```python
from build123d import *

# Parameters (mm, degrees)
SKETCH_1_W               = 198
SKETCH_1_H               = 30
EXTRUDE_1_DEPTH          = 2
HOLE_WIZARD_1_D          = 2.75
HOLE_WIZARD_1_DEPTH      = 100
CUT_EXTRUDE_1_DEPTH      = 101.149887668
CUT_EXTRUDE_1_DEPTH_BACK = 101.149887668


with BuildPart() as part:
    # 草图1 → 凸台-拉伸1 (new body)
    with BuildSketch(Plane(origin=(0, 0, 0), x_dir=(1, 0, 0), z_dir=(0, 1, 0))):
        Rectangle(SKETCH_1_W, SKETCH_1_H)
    extrude(amount=EXTRUDE_1_DEPTH)

    # 孔1
    with Locations(Plane(origin=(0, 2, 0), x_dir=(1, 0, 0), z_dir=(0, 1, 0))):
        with Locations((95, 10.999999819), (95, -11), (20.000000003, 10.999999819), (20.000000003, -11), (-95.2, 10.999999819), (-95.2, -11), (-20.200000003, 10.999999819), (-20.200000003, -11), (-34.700003407, -11), (-62.700003407, -11), (62.500003407, -11), (34.500003407, -11)):
            Hole(HOLE_WIZARD_1_D / 2, depth=HOLE_WIZARD_1_DEPTH)

    # 草图4 → 切除-拉伸1 (cut, two sides: drawn at the far end of the back side and taken through both)
    with BuildSketch(Plane(origin=(0, 2, 0), x_dir=(1, 0, 0), z_dir=(0, 1, 0)).offset(-CUT_EXTRUDE_1_DEPTH_BACK)):
        with BuildLine():
            Line((-10, 7), (10, 7))
            ThreePointArc((10, 7), (17, 0), (10, -7))
            Line((10, -7), (-10, -7))
            ThreePointArc((-10, -7), (-17, 0), (-10, 7))
        make_face()
        with BuildLine():
            Line((-84.999999997, 7), (-30.400000007, 7))
            ThreePointArc((-30.400000007, 7), (-23.400000007, 0), (-30.400000007, -7))
            Line((-30.400000007, -7), (-84.999999997, -7))
            ThreePointArc((-84.999999997, -7), (-91.999999997, 0), (-84.999999997, 7))
        make_face()
        with BuildLine():
            Line((84.999999997, 7), (30.400000007, 7))
            ThreePointArc((30.400000007, 7), (23.400000007, 0), (30.400000007, -7))
            Line((30.400000007, -7), (84.999999997, -7))
            ThreePointArc((84.999999997, -7), (91.999999997, 0), (84.999999997, 7))
        make_face()
    extrude(amount=CUT_EXTRUDE_1_DEPTH + CUT_EXTRUDE_1_DEPTH_BACK, mode=Mode.SUBTRACT)


solid = part.part
```
The model under review builds one solid part; all positions refer to its coordinate system, in mm. A direction names the side the tool comes from. Round coordinates to 2 decimals unless told otherwise and drop trailing zeros. Loops run counter-clockwise (first coordinate to the right, second up) from the corner with the lowest first, then second, coordinate; pieces in that order, holes last. Notation, with made-up numbers: M 37,-36 L 72,-36 A6 cw 72,-31 Z; hole C -5,-28 d1. An arc over 180 degrees is marked long. Write item = value, one per line.
Item 1: Machinability: for faces 3 (the cylindrical face through (17, 1, 0)), 4 (the flat face through (-1, 0, -10)), which of the approach directions +Z, -Z, +X, -X, +Y, -Y give a long, thin tool a straight path to every point of the face, cutting with its end or side? Answer none if there is none.
Return value:
face_3 = +Y, -Y
face_4 = +Z, -Z, +X, -X, -Y
Item 2: Take a section at B-B on y = 0.3. State how many separate pieces and enclosed holes the cut face has, then the cut area to 3 significant figures.
Return value:
separate_pieces = 1
enclosed_holes = 15
area = 3,600 mm2
Item 3: The part is to be moulded in two halves that separate along Z. For faces 1 (the flat face through (-1, 2, -10)), 2 (the cylindrical face through (92, 1, 0)), say which applies: released by +Z, released by -Z, zero draft, split by the parting line, or undercut.
Return value:
face_1 = zero draft
face_2 = undercut
Item 4: Take a section at C-C on x = -5. Write out the cut boundary in (y, z).
Return value:
outline = M 0,-15 L 2,-15 L 2,-7 L 0,-7 Z; M 0,7 L 2,7 L 2,15 L 0,15 Z
Item 5: Insertion check: P1, Ø2.5, axis at x = -34.7, z = 11, coming from the -Y side. The pin has a flat end and moves straight along its axis. Give the tip position at first contact, or say it passes through.
Return value:
P1 = through
Item 6: Take a section at A-A on z = 0. Write out the cut boundary in (x, y).
Return value:
outline = M -99,0 L -92,0 L -92,2 L -99,2 Z; M -23.4,0 L -17,0 L -17,2 L -23.4,2 Z; M 17,0 L 23.4,0 L 23.4,2 L 17,2 Z; M 92,0 L 99,0 L 99,2 L 92,2 Z
Item 7: For line 1 (Z direction, x = 81, y = 1.3); line 2 (Z direction, x = -20.2, y = 1.4) (3 decimals); line 3 (X direction, y = 1, z = -6.25), list the stretches that pass through material, from the lowest coordinate up. Write a range as [from, to].
Return value:
line_1 = [-15, -7], [7, 15]
line_2 = [-15, -12.375], [-9.625, 9.625], [12.375, 15]
line_3 = [-99, -88.15], [-27.25, -13.15], [13.15, 27.25], [88.15, 99]
